Part model, mm, in its own coordinate system. Round coordinates to 2 decimals unless told otherwise and drop trailing zeros. Write each loop counter-clockwise with the first axis right and the second up, starting at its lowest first coordinate (ties: lowest second). Pieces come first, ordered by that corner, then holes. Notation, with made-up numbers: (50.5, 8.25) -> (73.5, 8.25) arc R12 cw to (73.5, 12.25) -> close; hole circle Ø5 at (-33, -9). An arc over 180 degrees is marked (long way). Use CSV: the item, a comma, the result in double quotes. Start each with the question number.
(1) Probe line 1 (Y direction, x = 202, z = 4.75); line 2 (X direction, y = 314, z = 0.25); line 3 (Z direction, x = 234.5, y = 496). List the from-to ranges inside material, lowest first. Write a range as [from, to].
(2) Drop flat-ended pins along their axis: pin 1 (1 mm diameter, centred on y = 435.5, z = -2.5, fed in from -X); pin 2 (4 mm diameter, centred on x = 48.5, z = 0.5, fed in from -Y). Give the stop position or say it passes through.
(3) Saw through at A-A (y = 772.5). Give the cut face in (x, z).
(4) Saw through at C-C (x = 182.5). Give the cut face in (y, z).
(5) Saw through at B-B (z = -2.75). Give the cut face in (x, y).
```python
from build123d import *


with BuildPart() as part:
    # Sweep3: sweep along a path in Sketch2
    with BuildLine(Plane.XY) as sweep3_path:
        Line((0, 0), (0, 480))
        ThreePointArc((0, 480), (5.857864376, 494.142135624), (20, 500))
        Line((20, 500), (280, 500))
        ThreePointArc((280, 500), (294.142135624, 505.857864376), (300, 520))
        Line((300, 520), (300, 900))
    # Sketch3 → Sweep3 (sweep)
    with BuildSketch(Plane(origin=(0, 0, 0), x_dir=(1, 0, 0), z_dir=(0, 1, 0))):
        Polygon((2.886751346, 5), (-2.886751346, 5), (-5.773502692, 0), (-2.886751346, -5), (2.886751346, -5), (5.773502692, 0), align=None)
    sweep(path=sweep3_path.line)


solid = part.part
```
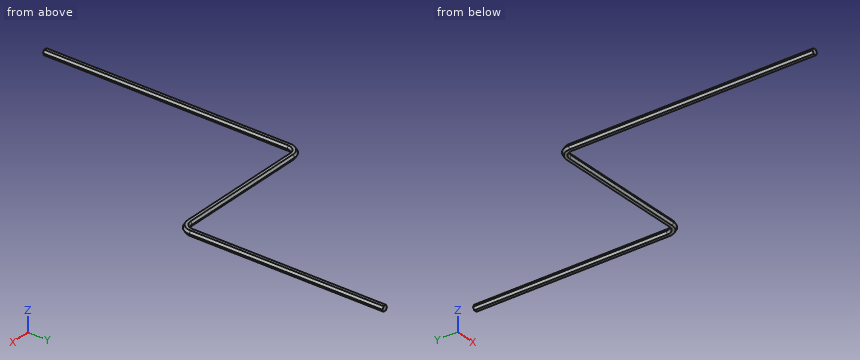
Answers:
1,line 1,"y = [496.97, 503.03]"
1,line 2,"x = [-5.63, 5.63]"
1,line 3,"z = [-3.07, 3.07]"
2,pin 1,"stops at x = -4.62"
2,pin 2,"stops at y = 494.23"
3,outline,"(294.23, 0) -> (297.11, -5) -> (302.89, -5) -> (305.77, 0) -> (302.89, 5) -> (297.11, 5) -> close"
4,outline,"(494.23, 0) -> (497.11, -5) -> (502.89, -5) -> (505.77, 0) -> (502.89, 5) -> (497.11, 5) -> close"
5,outline,"(-4.19, 0) -> (4.19, 0) -> (4.19, 480) arc R15.81 cw to (20, 495.81) -> (280, 495.81) arc R24.19 ccw to (304.19, 520) -> (304.19, 900) -> (295.81, 900) -> (295.81, 520) arc R15.81 cw to (280, 504.19) -> (20, 504.19) arc R24.19 ccw to (-4.19, 480) -> close"
